from build123d import *

# Parameters (mm, degrees)
SKETCH1_W                                        = 76.2
SKETCH1_H                                        = 127
SKETCH1_R                                        = 3.429
BOSS_EXTRUDE1_DEPTH                              = 12.7
CBORE_FOR_1_4_SOCKET_HEAD_CAP_SCREW1_D           = 6.7564
CBORE_FOR_1_4_SOCKET_HEAD_CAP_SCREW1_CBORE_D     = 11.1125
CBORE_FOR_1_4_SOCKET_HEAD_CAP_SCREW1_CBORE_DEPTH = 6.35
F_1_4_20_TAPPED_HOLE1_D                          = 5.1054


with BuildPart() as part:
    # Sketch1 → Boss-Extrude1 (new body)
    with BuildSketch(Plane(origin=(0, 0, 0), x_dir=(1, 0, 0), z_dir=(0, 1, 0))):
        Rectangle(SKETCH1_W, SKETCH1_H)
        with Locations(Location((-12.7, 12.7, 0), (0, 0, 270))):
            Circle(SKETCH1_R, mode=Mode.SUBTRACT)
        with Locations(Location((12.7, 12.7, 0), (0, 0, 270))):
            Circle(SKETCH1_R, mode=Mode.SUBTRACT)
        with Locations(Location((12.7, -12.7, 0), (0, 0, 270))):
            Circle(SKETCH1_R, mode=Mode.SUBTRACT)
        with Locations(Location((-12.7, -12.7, 0), (0, 0, 270))):
            Circle(SKETCH1_R, mode=Mode.SUBTRACT)
    extrude(amount=BOSS_EXTRUDE1_DEPTH)

    # CBORE for 1/4 Socket Head Cap Screw1 (through all)
    with Locations(Plane(origin=(0, 12.7, 0), x_dir=(1, 0, 0), z_dir=(0, 1, 0))):
        with Locations((-12.7, 12.7), (12.7, 12.7), (12.7, -12.7), (-12.7, -12.7), (-108.226831433, 58.259256328)):
            CounterBoreHole(CBORE_FOR_1_4_SOCKET_HEAD_CAP_SCREW1_D / 2, CBORE_FOR_1_4_SOCKET_HEAD_CAP_SCREW1_CBORE_D / 2, CBORE_FOR_1_4_SOCKET_HEAD_CAP_SCREW1_CBORE_DEPTH)

    # 1/4-20 Tapped Hole1 (through all)
    with Locations(Plane(origin=(0, 12.7, 0), x_dir=(1, 0, 0), z_dir=(0, 1, 0))):
        with Locations((25.4, 50.8), (-25.4, 50.8), (-25.4, -50.8), (25.4, -50.8)):
            Hole(F_1_4_20_TAPPED_HOLE1_D / 2)


solid = part.part
Work out the finished part from the listing and answer in its coordinate system (mm). A direction names the side the tool comes from. Round coordinates to 2 decimals unless told otherwise and drop trailing zeros. Write each loop counter-clockwise with the first axis right and the second up, starting at its lowest first coordinate (ties: lowest second). Pieces come first, ordered by that corner, then holes. Notation, with made-up numbers: (-0.5, 72) -> (44.5, 72) arc R10 ccw to (44.5, 83) -> close; hole circle Ø2 at (73.25, 25.5). An arc over 180 degrees is marked (long way). Write each question's results on one line, items separated by ' | '.
Item 1: Find the intervals of material crossed by line 1 along Z through (x, y) = (-12.7, 11.25); line 2 along Z through (x, y) = (-25.4, 8.5); line 3 along X through (y, z) = (9.25, -50.8), in increasing order. Write a range as [from, to].
Result set:
line 1: [-63.5, -18.26], [-7.14, 7.14], [18.26, 63.5] | line 2: [-63.5, -53.35], [-48.25, 48.25], [53.35, 63.5] | line 3: [-38.1, -27.95], [-22.85, 22.85], [27.95, 38.1]
Item 2: Flat-ended cylindrical pins translate along their axes: P1, Ø9, axis at x = 12.7, z = 12.7, coming from the +Y side; P2, Ø5.5, axis at x = -12.7, z = 12.7, coming from the -Y side. Find the tip coordinate at first contact, or state that the pin passes through.
Result set:
P1: y = 6.35 | P2: through
Item 3: The mould has two halves that part along X. Classify faces 1 (the face through (9.35, 3.13, 11.96)), 2 (the face through (-1, 0, -1)), 3 (the face through (-12.549, 3.131, 9.274)), 4 (the face through (-38.1, 6, 1)): +X half, -X half, draft (parallel to the pull), parting line (faces both ways), or undercut.
Result set:
face 1: undercut | face 2: draft | face 3: undercut | face 4: -X half
Item 4: A cutting plane is placed at A-A, the plane x = 12.7. Determine the outline of the cut face in (y, z).
Result set:
outline: (0, -63.5) -> (12.7, -63.5) -> (12.7, -18.26) -> (6.35, -18.26) -> (6.35, -16.13) -> (0, -16.13) -> close; (0, -9.27) -> (6.35, -9.27) -> (6.35, -7.14) -> (12.7, -7.14) -> (12.7, 7.14) -> (6.35, 7.14) -> (6.35, 9.27) -> (0, 9.27) -> close; (0, 16.13) -> (6.35, 16.13) -> (6.35, 18.26) -> (12.7, 18.26) -> (12.7, 63.5) -> (0, 63.5) -> close
Item 5: Which of the six approach directions +Z, -Z, +X, -X, +Y, -Y give full straight-line access (tool end or side, diameter ignored) to faces 5 (the face through (-1, 6, 63.5)), 6 (the face through (7.15, 9.57, -12.94))?
Result set:
face 5: +Z, +X, -X, +Y, -Y | face 6: +Y
Item 6: A cutting plane is placed at B-B, the plane z = -12.7. Determine the outline of the cut face in (x, y).
Result set:
outline: (-38.1, 0) -> (-16.13, 0) -> (-16.13, 6.35) -> (-18.26, 6.35) -> (-18.26, 12.7) -> (-38.1, 12.7) -> close; (-9.27, 0) -> (9.27, 0) -> (9.27, 6.35) -> (7.14, 6.35) -> (7.14, 12.7) -> (-7.14, 12.7) -> (-7.14, 6.35) -> (-9.27, 6.35) -> close; (16.13, 0) -> (38.1, 0) -> (38.1, 12.7) -> (18.26, 12.7) -> (18.26, 6.35) -> (16.13, 6.35) -> close
Item 7: A cutting plane is placed at C-C, the plane y = 9.5. Count the separate pieces of the cut face and the enclosed holes in it, plus the area to 3 significant figures.
Result set:
separate pieces: 1 | enclosed holes: 8 | area: 9,210 mm^2
Item 8: A cutting plane is placed at D-D, the plane z = -50.8. Determine the outline of the cut face in (x, y).
Result set:
outline: (-38.1, 0) -> (-27.95, 0) -> (-27.95, 12.7) -> (-38.1, 12.7) -> close; (-22.85, 0) -> (22.85, 0) -> (22.85, 12.7) -> (-22.85, 12.7) -> close; (27.95, 0) -> (38.1, 0) -> (38.1, 12.7) -> (27.95, 12.7) -> close
